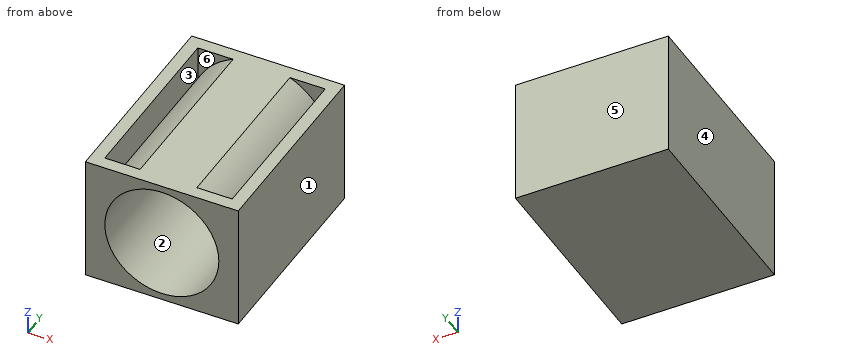
```python
from build123d import *

# Parameters (mm, degrees)
F0_W     = 30
F0_H     = 25
F1_DEPTH = 40
F2_R     = 11.1868683522
F3_DEPTH = 37
F4_T     = 2.5


# Not quite as in the source:
# - a shell that OpenCascade refuses in one call is made with other operations: the cavity is built on its own and cut out


with BuildPart() as f1:
    # F0 (on Front) → F1 (new body)
    with BuildSketch(Plane.XZ):
        Rectangle(F0_W, F0_H)
    extrude(amount=F1_DEPTH)

    # F2 (on face) → F3 (cut)
    with BuildSketch(Plane.XZ.offset(40)):
        Circle(F2_R)
    extrude(amount=-F3_DEPTH, mode=Mode.SUBTRACT)

    # F4: shell of thickness 2.5, made by hand


with BuildPart() as f4_core1:
    # F4_t2: copy of F1
    add(f1.part)

    # the walls: a layer under each face that stays
    f4_faces = [f4_core1.faces().sort_by_distance(p)[0] for p in [
        (0, -20, -12.5),
        (-15, -20, 0),
        (15, -20, 0),
        (0, 0, 0),
        (-10, -40, -8.3333333333),
        (-11.1868683522, -21.5, 0),
        (0, -3, 0),
    ]]
    thicken(f4_faces, amount=-F4_T, mode=Mode.SUBTRACT)

    # F4_s3 → F4_t4 (revolve, cut)
    with BuildSketch(Plane.XY):
        Polygon((11.1618683522, -3.025), (13.6868683522, -3), (13.6868683522, -0.5), (11.1868683522, -0.5), align=None)
    revolve(axis=Axis((0, -3, 0), (0, -1, 0)), mode=Mode.SUBTRACT)


with BuildPart() as f1_1:
    add(f1.part)

    # what is left inside the walls is the cavity
    f4_cavity = [f4_core1.part.solids().sort_by_distance(p)[0] for p in [
        (-9.695755, -25.833333, 9.695755),
        (9.695755, -25.833333, 9.695755),
        (11.164727, -25.833333, -7.960164),
        (-11.164727, -25.833333, -7.960164),
    ]]
    add(f4_cavity, mode=Mode.SUBTRACT)


solid = f1_1.part
```
Geometry check sheet. Reference: the model listing, model coordinates, mm. Face numbers are marked on the shaded views. A direction names the side the tool comes from. Coordinates: 2 decimals unless noted, no trailing zeros. Order: outer loops, then holes, each group sorted by start corner. A loop starts at its lowest first (then second) coordinate and runs counter-clockwise, first axis right, second up. Notation, with made-up numbers: M -29.5,-8 L -14.5,-8 A14 ccw -14.5,4 Z; hole C -40,-18.75 d5. An arc over 180 degrees is marked long. Answer as a JSON object with one key per item and string values.
Q1. Depth check by flat-ended pin: pin 1 Ø2.5 at (x, y) = (10.5, -22) entering from +Z; pin 2 Ø0.9 at (x, y) = (-11, -22.5) entering from +Z. Enter the tip coordinate at first touch or a pass-through.
Results are:
{"pin 1": "stops at z = 10.09", "pin 2": "stops at z = 8.72"}
Q2. Scan lines: line 1 (Z direction, x = 0, y = -19.5); line 2 (Y direction, x = -11.5, z = 10.75); line 3 (X direction, y = -8.5, z = -7.5). Record each from-to range of solid material in increasing order.
Results are:
{"line 1": "z = -12.5 to -11.19, 11.19 to 12.5", "line 2": "y = -40 to -37.5, -2.5 to 0", "line 3": "x = -15 to -12.5, -11.45 to -8.3, 8.3 to 11.45, 12.5 to 15"}
Q3. Cross-section at A-A on y = -16.5. Record the cut outline in (x, z).
Results are:
{"outline": "M -15,-12.5 L 15,-12.5 L 15,12.5 L 12.5,12.5 L 12.5,5.57 A13.69 ccw 5.57,12.5 L -5.57,12.5 A13.69 ccw -12.5,5.57 L -12.5,12.5 L -15,12.5 Z; hole M -12.5,-10 L -9.35,-10 A13.69 cw -12.5,-5.57 Z; hole C 0,0 d22.37; hole M 9.35,-10 L 12.5,-10 L 12.5,-5.57 A13.69 cw Z"}
Q4. Tool access check on the marked faces 1 and 2. Record the directions out of +Z, -Z, +X, -X, +Y, -Y that give a thin tool (end or side, any length) a straight path to the whole face; none if there is none.
Results are:
{"face 1": "+Z, -Z, +X, +Y, -Y", "face 2": "-Y"}
Q5. Cross-section at D-D on x = -12. Record the cut outline in (y, z).
Results are:
{"outline": "M -40,-12.5 L 0,-12.5 L 0,12.5 L -2.5,12.5 L -2.5,6.58 L -37.5,6.58 L -37.5,12.5 L -40,12.5 Z; hole M -37.5,-10 L -2.5,-10 L -2.5,-6.58 L -37.5,-6.58 Z"}
Q6. Cross-section at B-B on z = 10.5. Record the cut outline in (x, y).
Results are:
{"outline": "M -15,-40 L -3.86,-40 L -3.86,-3 L 3.86,-3 L 3.86,-40 L 15,-40 L 15,0 L -15,0 Z; hole M -12.5,-37.5 L -8.78,-37.5 L -8.78,-2.5 L -12.5,-2.5 Z; hole M 8.78,-37.5 L 12.5,-37.5 L 12.5,-2.5 L 8.78,-2.5 Z"}
Q7. Cross-section at C-C on x = 0. Record the cut outline in (y, z), and give its area (3 significant figures).
Results are:
{"outline": "M -40,-12.5 L 0,-12.5 L 0,12.5 L -40,12.5 L -40,11.19 L -3,11.19 L -3,-11.19 L -40,-11.19 Z", "area": "172 mm²"}
Q8. Release check for a two-part mould opening along Y. For the marked faces 3, 4, 5 and 6 record: released by +Y, released by -Y, zero draft, split by the parting line, or undercut.
Results are:
{"face 3": "undercut", "face 4": "zero draft", "face 5": "released by +Y", "face 6": "undercut"}
